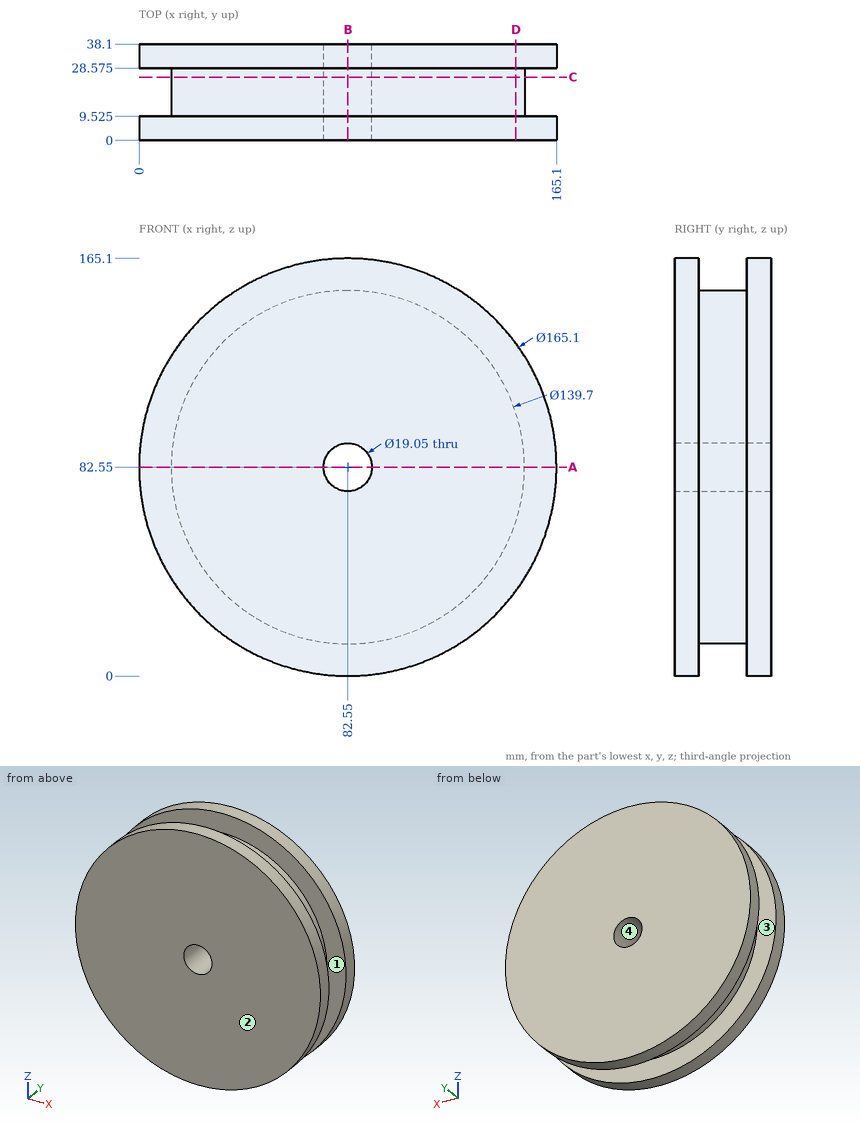
The figure shows three views and two pictorial views of one solid part (mm, origin at its lowest corner). Answer the questions. A direction names the side the tool comes from. Round coordinates to 2 decimals unless told otherwise and drop trailing zeros. Order: outer loops, then holes, each group sorted by start corner. A loop starts at its lowest first (then second) coordinate and runs counter-clockwise, first axis right, second up. Notation, with made-up numbers: (-8.5, 88.25) - (20.5, 88.25) arc R17 ccw to (20.5, 97.25) - close; hole circle Ø4 at (49, -7). An arc over 180 degrees is marked (long way). Write item = value, one per line. Start each with the question number.
1) Section A-A, the plane z = 82.55 is taken. Write down the section's boundary in (x, y) (3 decimals), plus the area to 3 significant figures.
2) For the marked faces 1 and 2, determine the directions among +Z, -Z, +X, -X, +Y, -Y from which every point of the face is accessible in a straight line to the end or side of a thin tool.
3) Section C-C, the plane y = 25 is taken. Write down the section's boundary in (x, z) (3 decimals).
4) Given pin 1 (4 mm diameter, centred on y = 29.5, z = 111, fed in from -X); pin 2 (10 mm diameter, centred on x = 78.5, z = 76, fed in from +Y); pin 3 (6 mm diameter, centred on x = 24, y = 22, fed in from +Z); pin 4 (2 mm diameter, centred on y = 8.5, z = 63, fed in from +X), each flat-ended and moving along its own axis, determine where each tip first touches the part or whether it passes through.
5) Straight lines are drawn through the part: L1, parallel to Z at x = 82, y = 21; L2, parallel to Y at x = 151.5, z = 127.5 (3 decimals). For each, find the intervals that lie inside material, in ascending order.
6) For a pull along X with two mould halves and no side action, classify the marked faces 3 and 4 as released by +X, released by -X, zero draft, split by the parting line, or undercut.
7) Section B-B, the plane x = 82.55 is taken. Write down the section's boundary in (y, z) (3 decimals).
8) Section D-D, the plane x = 149 is taken. Write down the section's boundary in (y, z) (3 decimals).
Results list:
q1.outline = (0, 0) - (73.025, 0) - (73.025, 38.1) - (0, 38.1) - (0, 28.575) - (12.7, 28.575) - (12.7, 9.525) - (0, 9.525) - close; (92.075, 0) - (165.1, 0) - (165.1, 9.525) - (152.4, 9.525) - (152.4, 28.575) - (165.1, 28.575) - (165.1, 38.1) - (92.075, 38.1) - close
q1.area = 5,080 mm^2
q2.face_1 = none
q2.face_2 = +Z, -Z, +X, -X, -Y
q3.outline = circle Ø139.7 at (82.55, 82.55); hole circle Ø19.05 at (82.55, 82.55)
q4.pin_1 = 4.35
q4.pin_2 = 38.1
q4.pin_3 = 124.9
q4.pin_4 = 162.99
q5.L1 = 12.7 to 73.04, 92.06 to 152.4
q5.L2 = 0 to 9.525, 28.575 to 38.1
q6.face_3 = zero draft
q6.face_4 = undercut
q7.outline = (0, 0) - (9.525, 0) - (9.525, 12.7) - (28.575, 12.7) - (28.575, 0) - (38.1, 0) - (38.1, 73.025) - (0, 73.025) - close; (0, 92.075) - (38.1, 92.075) - (38.1, 165.1) - (28.575, 165.1) - (28.575, 152.4) - (9.525, 152.4) - (9.525, 165.1) - (0, 165.1) - close
q8.outline = (0, 33.571) - (9.525, 33.571) - (9.525, 61.023) - (28.575, 61.023) - (28.575, 33.571) - (38.1, 33.571) - (38.1, 131.529) - (28.575, 131.529) - (28.575, 104.077) - (9.525, 104.077) - (9.525, 131.529) - (0, 131.529) - close
